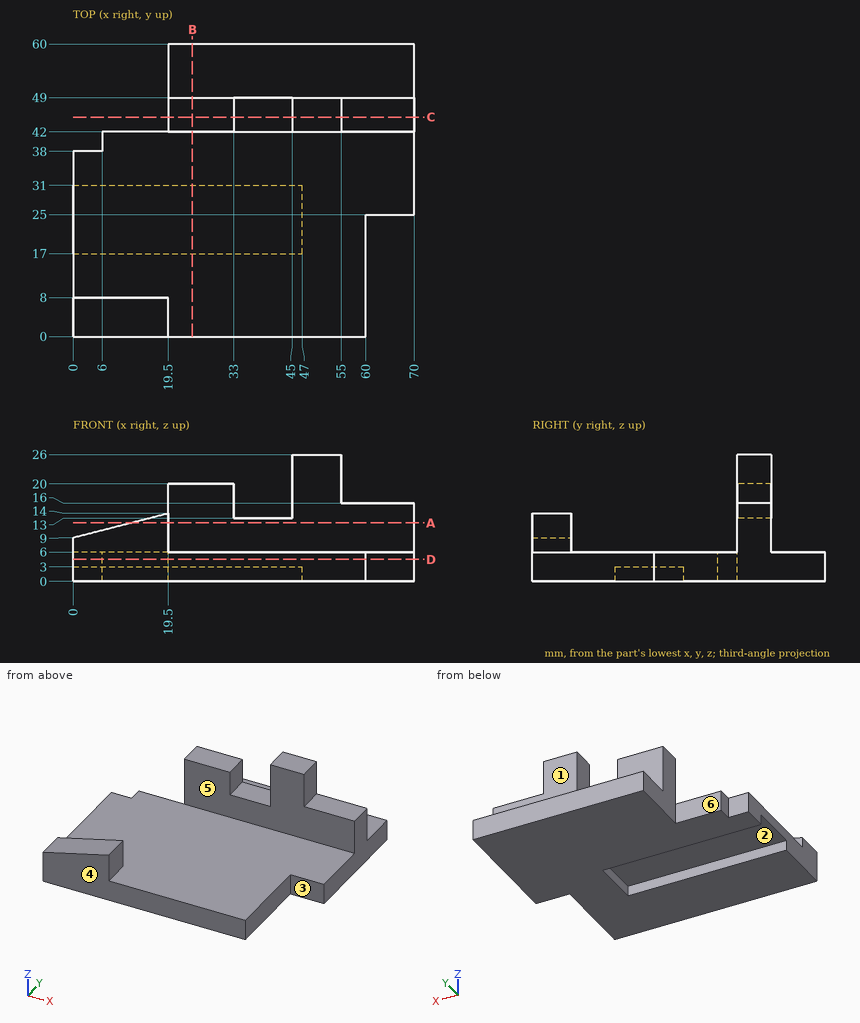
Design review of the part shown in the three views and the two pictorial views. Dimensions are in mm from the part's minimum x, y and z. A direction names the side the tool comes from. Give positions to 0.01 mm unless a question says otherwise; leave off trailing zeros. Loops run counter-clockwise (first coordinate to the right, second up) from the corner with the lowest first, then second, coordinate; pieces in that order, holes last. Notation, with made-up numbers: M 44.25,-22.75 L 82.25,-22.75 A11 cw 82.25,-2.75 Z; hole C 85.25,27 d10. An arc over 180 degrees is marked long. Put each result on its own line as item: value. Start each with the question number.
(1) Wall thickness on L1, parallel to Z at x = 22.5, y = 19.5; L2, parallel to Y at x = 46.5, z = 17; L3, parallel to Z at x = 58.5, y = 26.5: over which ranges is each line inside the solid? List them lowest first.
(2) Add section B-B, the plane x = 24.5. Write out the cut boundary in (y, z).
(3) For pin 1 (4 mm diameter, centred on x = 13.5, z = 7.5, fed in from +Y); pin 2 (0.9 mm diameter, centred on y = 21.5, z = 1, fed in from -X); pin 3 (7.5 mm diameter, centred on x = 61, y = 45, fed in from +Z); pin 4 (2.5 mm diameter, centred on x = 17, z = 1, fed in from -Y), all flat-tipped, find the tip position at first contact; note any pin that passes through.
(4) The part is to be moulded in two halves that separate along Y. For the marked faces 1, 2 and 3, say which applies: +Y half, -Y half, draft (parallel to the pull), parting line (faces both ways), or undercut.
(5) Add section D-D, the plane z = 4.5. Write out the cut boundary in (x, y).
(6) Add section C-C, the plane y = 45. Write out the cut boundary in (x, z).
(7) Machinability: for the marked faces 4, 5 and 6, which of the approach directions +Z, -Z, +X, -X, +Y, -Y give a long, thin tool a straight path to every point of the face, cutting with its end or side? Answer none if there is none.
(8) Add section A-A, the plane z = 12. Write out the cut boundary in (x, y).
Result:
1. L1: z = 3 to 6
1. L2: y = 42 to 49
1. L3: z = 0 to 6
2. outline: M 0,0 L 17,0 L 17,3 L 31,3 L 31,0 L 60,0 L 60,6 L 49,6 L 49,20 L 42,20 L 42,6 L 0,6 Z
3. pin 1: stops at y = 42
3. pin 2: stops at x = 47
3. pin 3: stops at z = 16
3. pin 4: stops at y = 0
4. face 1: +Y half
4. face 2: undercut
4. face 3: -Y half
5. outline: M 0,0 L 60,0 L 60,25 L 70,25 L 70,60 L 19.5,60 L 19.5,42 L 6,42 L 6,38 L 0,38 Z
6. outline: M 19.5,0 L 70,0 L 70,16 L 55,16 L 55,26 L 45,26 L 45,13 L 33,13 L 33,20 L 19.5,20 Z
7. face 4: +Z, -Z, +X, -X, -Y
7. face 5: +Z, +X, -X, -Y
7. face 6: +Z, -Z, -X, +Y
8. outline: M 11.7,0 L 19.5,0 L 19.5,8 L 11.7,8 Z; M 19.5,42 L 70,42 L 70,49 L 19.5,49 Z
